Verification items for the finished model (mm, model axes). A direction names the side the tool comes from. Coordinates: 2 decimals unless noted, no trailing zeros. Loops run counter-clockwise (first coordinate to the right, second up) from the corner with the lowest first, then second, coordinate; pieces in that order, holes last.
Q1. Go/stop test with a flat-tipped pin: P1, Ø3, axis at x = 24.5, z = -77.5, coming from the +Y side (3 decimals). Record where the tip stops, or that it passes through.
Q2. Sectioned sample at B-B (y = -16.5). Enter the section's corners in (x, z) (3 decimals).
Q3. Mould release check, pull along Y, two halves, no side actions. Record for faces 1 (the face through (0, 34.925, 47)), 2 (the face through (-1, 38.1, 47)), 3 (the face through (-3, -37, 200)): +Y half, -Y half, draft (parallel to the pull), parting line (faces both ways), or undercut.
Q4. Sectioned sample at D-D (z = -162). Enter the section's corners in (x, y) (3 decimals).
Q5. Material ranges on probe 1 along Z at (x, y) = (-31, 36); probe 2 along Y at (x, z) = (-36.15, 188); probe 3 along Y at (x, z) = (-17.5, -144.5) (3 decimals), recorded low to high.
Q6. Sectioned sample at A-A (x = 0). Enter the section's corners in (y, z) (3 decimals), then the cut area to 3 significant figures.
Q7. Access from +Z, -Z, +X, -X, +Y, -Y to the whole of each face (thin tool, end or side, straight path). Record for faces 4 (the face through (-3, -37, -200)), 5 (the face through (-34.925, 0, 3)).
Q8. Sectioned sample at C-C (z = 22). Enter the section's corners in (x, y) (3 decimals), then the cut area to 3 significant figures.
```python
from build123d import *

# Parameters (mm, degrees)
SKETCH1_W           = 76.2
SKETCH1_H           = 76.2
SKETCH1_W_2         = 69.85
SKETCH1_H_2         = 69.85
BOSS_EXTRUDE1_DEPTH = 200
SKETCH4_R           = 3.1
CUT_EXTRUDE2_DEPTH  = 218.389167163
CUT_EXTRUDE3_REACH  = 219.389
SKETCH5_R           = 2.1
SKETCH5_W           = 57.4
SKETCH5_H           = 57.4
FILLET1_R           = 2
SKETCH6_R           = 21.1
CUT_EXTRUDE4_DEPTH  = 218.389167163


with BuildPart() as part:
    # Sketch1 → Boss-Extrude1 (new, symmetric)
    with BuildSketch(Plane.XY):
        Rectangle(SKETCH1_W, SKETCH1_H)
        Rectangle(SKETCH1_W_2, SKETCH1_H_2, mode=Mode.SUBTRACT)
    extrude(amount=BOSS_EXTRUDE1_DEPTH, both=True)

    # Sketch4 → Cut-Extrude2 (cut, through all)
    with BuildSketch(Plane(origin=(38.1, 0, 0), x_dir=(0, 0, -1), z_dir=(1, 0, 0))):
        with Locations((-140, 24)):
            Circle(SKETCH4_R)
        with Locations((-188, 24)):
            Circle(SKETCH4_R)
        with Locations((-140, -24)):
            Circle(SKETCH4_R)
        with Locations((-188, -24)):
            Circle(SKETCH4_R)
    extrude(amount=-CUT_EXTRUDE2_DEPTH, mode=Mode.SUBTRACT)

    # Sketch5 → Cut-Extrude3 (cut, up to next)
    with BuildSketch(Plane(origin=(0, 38.1, 0), x_dir=(1, 0, 0), z_dir=(0, 1, 0)), mode=Mode.PRIVATE) as cut_extrude3_sk1:
        with Locations(Location((31, 38, 0), (0, 0, 180))):
            Circle(SKETCH5_R)
    cut_extrude3_tool1 = extrude(cut_extrude3_sk1.sketch, amount=-CUT_EXTRUDE3_REACH, mode=Mode.PRIVATE) & part.part
    # Sketch5 → Cut-Extrude3 (cut, up to next)
    with BuildSketch(Plane(origin=(0, 38.1, 0), x_dir=(1, 0, 0), z_dir=(0, 1, 0)), mode=Mode.PRIVATE) as cut_extrude3_sk2:
        with Locations(Location((-31, 100, 0), (0, 0, 180))):
            Circle(SKETCH5_R)
    cut_extrude3_tool2 = extrude(cut_extrude3_sk2.sketch, amount=-CUT_EXTRUDE3_REACH, mode=Mode.PRIVATE) & part.part
    # Sketch5 → Cut-Extrude3 (cut, up to next)
    with BuildSketch(Plane(origin=(0, 38.1, 0), x_dir=(1, 0, 0), z_dir=(0, 1, 0)), mode=Mode.PRIVATE) as cut_extrude3_sk3:
        with Locations(Location((-31, 38, 0), (0, 0, 180))):
            Circle(SKETCH5_R)
    cut_extrude3_tool3 = extrude(cut_extrude3_sk3.sketch, amount=-CUT_EXTRUDE3_REACH, mode=Mode.PRIVATE) & part.part
    # Sketch5 → Cut-Extrude3 (cut, up to next)
    with BuildSketch(Plane(origin=(0, 38.1, 0), x_dir=(1, 0, 0), z_dir=(0, 1, 0)), mode=Mode.PRIVATE) as cut_extrude3_sk4:
        with Locations(Location((31, 100, 0), (0, 0, 180))):
            Circle(SKETCH5_R)
    cut_extrude3_tool4 = extrude(cut_extrude3_sk4.sketch, amount=-CUT_EXTRUDE3_REACH, mode=Mode.PRIVATE) & part.part
    # Sketch5 → Cut-Extrude3 (cut, up to next)
    with BuildSketch(Plane(origin=(0, 38.1, 0), x_dir=(1, 0, 0), z_dir=(0, 1, 0)), mode=Mode.PRIVATE) as cut_extrude3_sk5:
        with Locations((0, 69)):
            Rectangle(SKETCH5_W, SKETCH5_H)
    cut_extrude3_tool5 = extrude(cut_extrude3_sk5.sketch, amount=-CUT_EXTRUDE3_REACH, mode=Mode.PRIVATE) & part.part
    add(cut_extrude3_tool1.solids().sort_by_distance((31, 38.1, -38))[0], mode=Mode.SUBTRACT)
    add(cut_extrude3_tool2.solids().sort_by_distance((-31, 38.1, -100))[0], mode=Mode.SUBTRACT)
    add(cut_extrude3_tool3.solids().sort_by_distance((-31, 38.1, -38))[0], mode=Mode.SUBTRACT)
    add(cut_extrude3_tool4.solids().sort_by_distance((31, 38.1, -100))[0], mode=Mode.SUBTRACT)
    add(cut_extrude3_tool5.solids().sort_by_distance((0, 38.1, -69))[0], mode=Mode.SUBTRACT)

    # Fillet1
    fillet1_edges = [part.edges().sort_by_distance(p)[0] for p in [
        (28.7, 36.5125, -97.7),
        (-28.7, 36.5125, -97.7),
        (-28.7, 36.5125, -40.3),
        (28.7, 36.5125, -40.3),
    ]]
    fillet(fillet1_edges, radius=FILLET1_R)

    # Sketch6 → Cut-Extrude4 (cut, through all)
    with BuildSketch(Plane(origin=(0, 38.1, 0), x_dir=(1, 0, 0), z_dir=(0, 1, 0))):
        with Locations(Location((0, 162, 0), (0, 0, 180))):
            Circle(SKETCH6_R)
    extrude(amount=-CUT_EXTRUDE4_DEPTH, mode=Mode.SUBTRACT)


solid = part.part
```
Geometry check:
1. P1: stops at y = -34.925
2. outline: (-38.1, -200) - (-34.925, -200) - (-34.925, 200) - (-38.1, 200) - close; (34.925, -200) - (38.1, -200) - (38.1, 200) - (34.925, 200) - close
3. face 1: undercut
3. face 2: +Y half
3. face 3: draft
4. outline: (-38.1, -38.1) - (-21.1, -38.1) - (-21.1, -34.925) - (-34.925, -34.925) - (-34.925, 34.925) - (-21.1, 34.925) - (-21.1, 38.1) - (-38.1, 38.1) - close; (21.1, -38.1) - (38.1, -38.1) - (38.1, 38.1) - (21.1, 38.1) - (21.1, 34.925) - (34.925, 34.925) - (34.925, -34.925) - (21.1, -34.925) - close
5. probe 1: z = -200 to -102.1, -97.9 to -40.1, -35.9 to 200
5. probe 2: y = -38.1 to -27.1, -20.9 to 20.9, 27.1 to 38.1
5. probe 3: y = -38.1 to -34.925, 34.925 to 38.1
6. outline: (-38.1, -200) - (-34.925, -200) - (-34.925, -183.1) - (-38.1, -183.1) - close; (-38.1, -140.9) - (-34.925, -140.9) - (-34.925, 200) - (-38.1, 200) - close; (34.925, -200) - (38.1, -200) - (38.1, -183.1) - (34.925, -183.1) - close; (34.925, -140.9) - (38.1, -140.9) - (38.1, -97.7) - (34.925, -97.7) - close; (34.925, -40.3) - (38.1, -40.3) - (38.1, 200) - (34.925, 200) - close
6. area: 2,090 mm2
7. face 4: -Z, +X, -X, +Y, -Y
7. face 5: +Z, -Z
8. outline: (-38.1, -38.1) - (38.1, -38.1) - (38.1, 38.1) - (-38.1, 38.1) - close; hole (-34.925, -34.925) - (34.925, -34.925) - (34.925, 34.925) - (-34.925, 34.925) - close
8. area: 927 mm2
